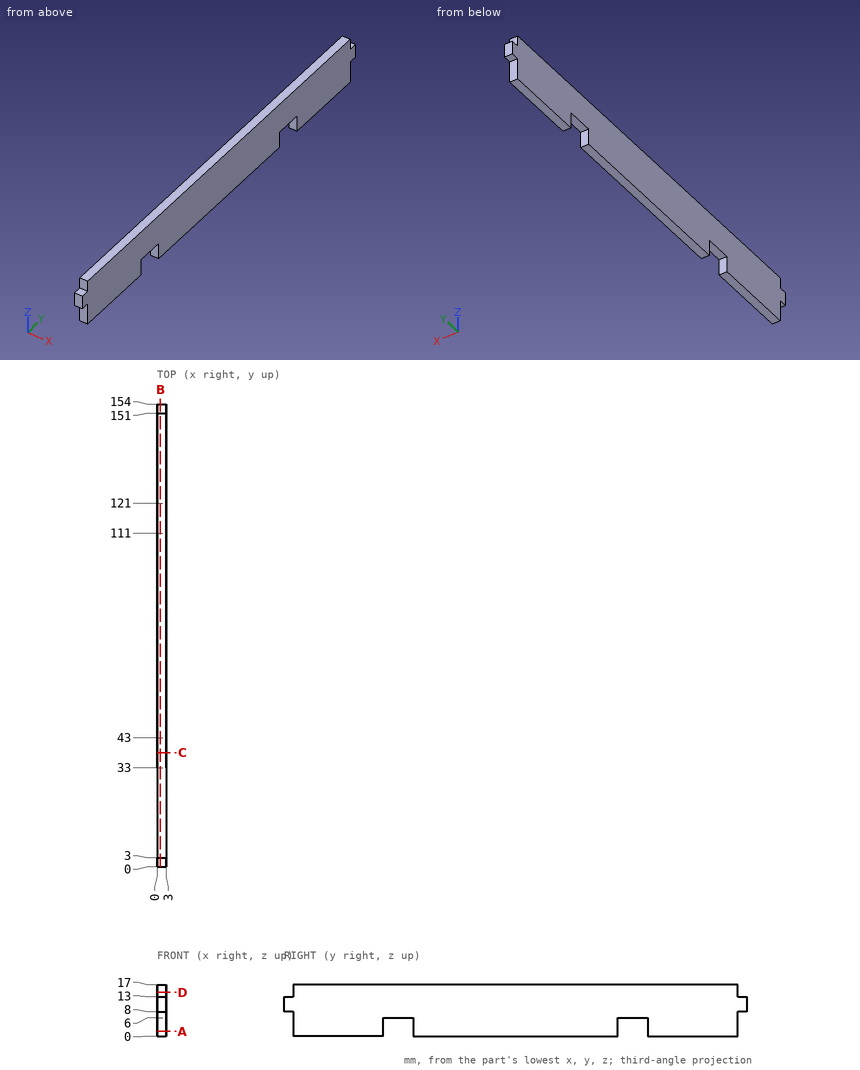
Part print with two shaded views. Sizes in mm from the minimum x, y, z corner. Round coordinates to 2 decimals unless told otherwise and drop trailing zeros. Loops run counter-clockwise (first coordinate to the right, second up) from the corner with the lowest first, then second, coordinate; pieces in that order, holes last. Notation, with made-up numbers: (69.25, 3.25) - (86.25, 3.25) arc R26 ccw to (86.25, 39.25) - close; hole circle Ø7 at (38, 82.5). An arc over 180 degrees is marked (long way). Put each result on its own line as item: value.
1. Slice it at D-D on z = 14.5. List the corners of the cut face in (x, y), and give its area (3 significant figures).
Geometry check:
outline: (0, 3) - (3, 3) - (3, 151) - (0, 151) - close
area: 444 mm²
2. Wall check: line 1 (Y direction, x = 2.1, z = 5.5); line 2 (Y direction, x = 2.2, z = 13.5); line 3 (Z direction, x = 2.4, y = 35). Give the ranges that are in metal, low to high.
Geometry check:
line 1: 3 to 33, 43 to 111, 121 to 151
line 2: 3 to 151
line 3: 6 to 17
3. Slice it at B-B on x = 1.1. List the corners of the cut face in (y, z).
Geometry check:
outline: (0, 8) - (3, 8) - (3, 0) - (33, 0) - (33, 6) - (43, 6) - (43, 0) - (111, 0) - (111, 6) - (121, 6) - (121, 0) - (151, 0) - (151, 8) - (154, 8) - (154, 13) - (151, 13) - (151, 17) - (3, 17) - (3, 13) - (0, 13) - close
4. Pin check, flat tips, straight feed: P1, Ø1.5, axis at x = 2, z = 3, coming from the +Y side; P2, Ø1.5, axis at x = 1.5, y = 153, coming from the -Z side; P3, Ø0.9, axis at x = 2, y = 152.5, coming from the +Z side. Stop position of each tip, or through.
Geometry check:
P1: y = 151
P2: z = 8
P3: z = 13
5. Slice it at C-C on y = 38. List the corners of the cut face in (x, z), and give its area (3 significant figures).
Geometry check:
outline: (0, 6) - (3, 6) - (3, 17) - (0, 17) - close
area: 33.0 mm²
6. Slice it at A-A on z = 1.5. List the corners of the cut face in (x, y).
Geometry check:
outline: (0, 3) - (3, 3) - (3, 33) - (0, 33) - close; (0, 43) - (3, 43) - (3, 111) - (0, 111) - close; (0, 121) - (3, 121) - (3, 151) - (0, 151) - close
